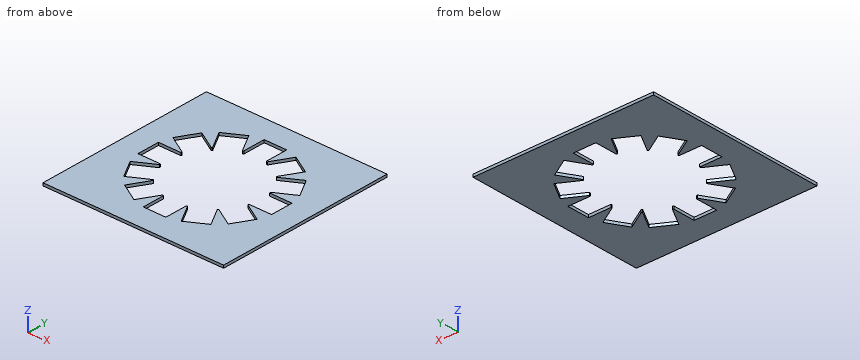
from build123d import *

# Parameters (mm, degrees)
SKETCH_W           = 399.99
SKETCH_H           = 399.99
PAD_DEPTH          = 6
SKETCH002_W        = 50
SKETCH002_H        = 50
POCKET001_DEPTH    = 1137.407205
POLARPATTERN_COUNT = 12
SKETCH003_R        = 101.355603
POCKET_DEPTH       = 6.001


with BuildPart() as part:
    # Sketch → Pad (new body)
    with BuildSketch(Plane.XY):
        Rectangle(SKETCH_W, SKETCH_H)
    extrude(amount=PAD_DEPTH)

    # Sketch002 → Pocket001 (cut, through all)
    with BuildSketch(Plane.XY.offset(6)):
        with Locations((0, 122.901995)):
            Rectangle(SKETCH002_W, SKETCH002_H)
    pocket001 = extrude(amount=-POCKET001_DEPTH, mode=Mode.SUBTRACT)

    # PolarPattern: Pocket001 ×12 about axis
    polarpattern_axis = Axis((0, 0, 6), (0, 0, 1))
    for i in range(1, POLARPATTERN_COUNT):
        add(pocket001.rotate(polarpattern_axis, i * 360 / POLARPATTERN_COUNT), mode=Mode.SUBTRACT)

    # Sketch003 → Pocket (cut, through all)
    with BuildSketch(Plane(origin=(0, 0, 0), x_dir=(-1, 0, 0), z_dir=(0, 0, -1))):
        Circle(SKETCH003_R)
    extrude(amount=-POCKET_DEPTH, mode=Mode.SUBTRACT)


solid = part.part
Geometry: final body of the model. Coordinates: model frame, mm. Coordinates: 2 decimals unless noted, no trailing zeros. Order: outer loops, then holes, each group sorted by start corner. A loop starts at its lowest first (then second) coordinate and runs counter-clockwise, first axis right, second up.
(1) Section query B-B (x = -131). Return the cut outline in (y, z) (3 decimals), plus the area to 3 significant figures.
(2) Material intervals for probe 1 along Y at (x, z) = (-143.5, 3) (3 decimals); probe 2 along X at (y, z) = (128, 2.25) (3 decimals); probe 3 along Y at (x, z) = (-84, 3.25) (3 decimals), sorted ascending.
(3) Section query A-A (y = -105). Return the cut outline in (x, z) (3 decimals).
(4) Section query C-C (x = 66). Return the cut outline in (y, z) (3 decimals), plus the area to 3 significant figures.
(5) Section query D-D (y = 60). Return the cut outline in (x, z) (1 decimal), plus the area to 3 significant figures.
Solution:
1. outline: (-199.995, 0) - (-68.905, 0) - (-68.905, 6) - (-199.995, 6) - close; (-46.765, 0) - (-25, 0) - (-25, 6) - (-46.765, 6) - close; (25, 0) - (46.765, 0) - (46.765, 6) - (25, 6) - close; (68.905, 0) - (199.995, 0) - (199.995, 6) - (68.905, 6) - close
1. area: 1,830 mm2
2. probe 1: y = -199.995 to -25, 25 to 199.995
2. probe 2: x = -199.995 to -74.101, -45.033 to -25, 25 to 45.033, 74.101 to 199.995
2. probe 3: y = -199.995 to -122.285, -95.492 to -77.365, 77.365 to 95.492, 122.285 to 199.995
3. outline: (-199.995, 0) - (-89.489, 0) - (-89.489, 6) - (-199.995, 6) - close; (-31.754, 0) - (-25, 0) - (-25, 6) - (-31.754, 6) - close; (25, 0) - (31.754, 0) - (31.754, 6) - (25, 6) - close; (89.489, 0) - (199.995, 0) - (199.995, 6) - (89.489, 6) - close
4. outline: (-199.995, 0) - (-132.677, 0) - (-132.677, 6) - (-199.995, 6) - close; (132.677, 0) - (199.995, 0) - (199.995, 6) - (132.677, 6) - close
4. area: 808 mm2
5. outline: (-200, 0) - (-136.1, 0) - (-136.1, 6) - (-200, 6) - close; (136.1, 0) - (200, 0) - (200, 6) - (136.1, 6) - close
5. area: 766 mm2
